Input: part model. Units: mm. Frame: model coordinates. Round coordinates to 2 decimals unless told otherwise and drop trailing zeros. Order: outer loops, then holes, each group sorted by start corner. A loop starts at its lowest first (then second) coordinate and runs counter-clockwise, first axis right, second up.
Item 1: Cut plane B-B on z = -110. Output: boundary loops of the cut face in (x, y).
Item 2: Cut plane C-C on x = 1.05. Output: boundary loops of the cut face in (y, z).
Item 3: Line query: L1, parallel to Z at x = 1.3, y = 97.5; L2, parallel to Y at x = 1.3, z = -113; L3, parallel to Z at x = 2.45, y = 53.5. Output: solid intervals per line, ascending.
Item 4: Cut plane A-A on y = 68. Output: boundary loops of the cut face in (x, z), then the cut area to 3 significant figures.
Autodesk Inventor part; units mm, degrees
ref_plane "YZ Plane" through (0, 0, 0) normal (1, 0, 0) x (0, 1, 0)
ref_plane "XZ Plane" through (0, 0, 0) normal (0, 1, 0) x (-1, 0, 0)
ref_plane "XY Plane" through (0, 0, 0) normal (0, 0, 1) x (1, 0, 0)
sketch "Sketch1" plane through (0, 0, 0) normal (1, 0, 0) x (0, 1, 0)
  line L0 (-114.3, 300.99) -> (114.3, 300.99)
  line L1 (114.3, 300.99) -> (114.3, -300.99)
  line L2 (114.3, -300.99) -> (-114.3, -300.99)
  line L3 (-114.3, -300.99) -> (-114.3, 300.99)
  line L4 (-114.3, 300.99) -> (114.3, -300.99) construction
  line L5 (114.3, 300.99) -> (-114.3, -300.99) construction
  point P0 (0, 0)
  dimension "d3" = 228.6
  dimension "d4" = 601.98
extrude "Extrusion2" add sketch "Sketch1" along normal blind 2.8575
fillet "Fillet1" radius 10.16 4 edges at (1.4287, -114.3, -300.99) (1.4287, 114.3, -300.99) (1.4287, -114.3, 300.99) (1.4287, 114.3, 300.99)
fillet "Fillet2" radius 0.5715 16 edges at (2.8575, 111.3242, 298.0142) (2.8575, 0, 300.99) (2.8575, -111.3242, 298.0142) (2.8575, -114.3, 0) (2.8575, -111.3242, -298.0142) (2.8575, 0, -300.99) (2.8575, 111.3242, -298.0142) (2.8575, 114.3, 0) (0, 111.3242, -298.0142) (0, 0, -300.99) (0, -111.3242, -298.0142) (0, -114.3, 0) (0, -111.3242, 298.0142) (0, 0, 300.99) (0, 111.3242, 298.0142) (0, 114.3, 0)
sketch "Sketch3" plane through (0, 0, 0) normal (-1, 0, 0) x (0, 0, 1)
  line L0 (300.4185, 104.14) -> (300.4185, -104.14)
  line L1 (290.83, -113.7285) -> (-290.83, -113.7285)
  line L2 (-290.83, 113.7285) -> (290.83, 113.7285)
  line L3 (-300.4185, -104.14) -> (-300.4185, 104.14)
  line L4 (290.83, 113.7285) -> (-290.83, 113.7285)
  line L5 (-97.2185, 125.0999) -> (-97.2185, 80.4789)
  line L6 (-97.2185, 80.4789) -> (-198.8185, 80.4789)
  line L7 (-198.8185, 80.4789) -> (-198.8185, 125.0999)
  line L8 (-97.2185, 125.0999) -> (-198.8185, 125.0999)
  line L9 (23.4315, 116.2685) -> (-14.6685, 116.2685)
  line L10 (-14.6685, 116.2685) -> (-14.6685, 59.1185)
  line L11 (-14.6685, 59.1185) -> (23.4315, 59.1185)
  line L12 (23.4315, 59.1185) -> (23.4315, 116.2685)
  dimension "d48" = 101.6
  dimension "d49" = 101.6
  dimension "d50" = 0
  dimension "d63" = 11.3714
  dimension "d64" = 33.2496
  dimension "d65" = 38.1
  dimension "d66" = 82.55
  dimension "d67" = 57.15
  dimension "d68" = 2.54
extrude "Extrusion3" cut sketch "Sketch3" against normal blind 5.08
sketch "Sketch4" plane through (2.8575, 0, 0) normal (1, 0, 0) x (0, 0, -1)
  circle A0 centre (234.3785, 106.1085) radius 2.54
  circle A1 centre (262.3185, 106.1085) radius 2.54
  line L0 (-290.83, 113.7285) -> (290.83, 113.7285)
  line L1 (300.4185, 104.14) -> (300.4185, -104.14)
  circle A2 centre (-262.89, 106.1085) radius 2.54
  circle A3 centre (-234.95, 106.1085) radius 2.54
  line L2 (-300.99, 104.14) -> (-300.99, -104.14)
  point P0 (0, 0)
  point P1 (198.8185, 113.7285)
  dimension "d52" = 5.08
  dimension "d53" = 7.62
  dimension "d54" = 27.94
  dimension "d55" = 38.1
  dimension "d58" = 27.94
  dimension "d60" = 38.1
extrude "Extrusion5" cut sketch "Sketch4" against normal up to next
equation "\"d58\" = d54"
equation "\"d60\" = d55"
equation "\"d61\" = d54"
properties part number "SideFlap2"
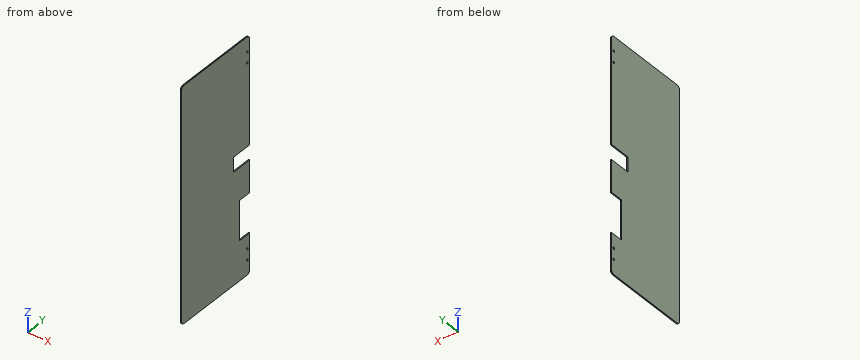
From the geometry:
1. outline: (0, -113.73) arc R0.57 ccw to (0.57, -114.3) - (2.29, -114.3) arc R0.57 ccw to (2.86, -113.73) - (2.86, 80.48) - (0, 80.48) - close
2. outline: (-114.3, -290.83) arc R10.16 ccw to (-104.14, -300.99) - (104.14, -300.99) arc R10.16 ccw to (114.3, -290.83) - (114.3, -198.82) - (80.48, -198.82) - (80.48, -97.22) - (114.3, -97.22) - (114.3, -14.67) - (59.12, -14.67) - (59.12, 23.43) - (114.3, 23.43) - (114.3, 290.83) arc R10.16 ccw to (104.14, 300.99) - (-104.14, 300.99) arc R10.16 ccw to (-114.3, 290.83) - close; hole circle Ø5.08 at (106.11, -262.32); hole circle Ø5.08 at (106.11, -234.38); hole circle Ø5.08 at (106.11, 234.95); hole circle Ø5.08 at (106.11, 262.89)
3. L1: z = -300.99 to -198.82, -97.22 to -14.67, 23.43 to 300.99
3. L2: y = -114.3 to 80.48
3. L3: z = -300.97 to 300.97
4. outline: (0, -300.42) arc R0.57 ccw to (0.57, -300.99) - (2.29, -300.99) arc R0.57 ccw to (2.86, -300.42) - (2.86, -14.67) - (0, -14.67) - close; (0, 23.43) - (2.86, 23.43) - (2.86, 300.42) arc R0.57 ccw to (2.29, 300.99) - (0.57, 300.99) arc R0.57 ccw to (0, 300.42) - close
4. area: 1,610 mm2
